Verification items for the finished model (mm, model axes). Face numbers are marked on the shaded views. Coordinates: 2 decimals unless noted, no trailing zeros. Loops run counter-clockwise (first coordinate to the right, second up) from the corner with the lowest first, then second, coordinate; pieces in that order, holes last. Notation, with made-up numbers: M 24.25,38 L 67.25,38 A31 ccw 67.25,62 Z; hole C 10.25,19.25 d6. An arc over 180 degrees is marked long. Write item = value, one per line. Start each with the question number.
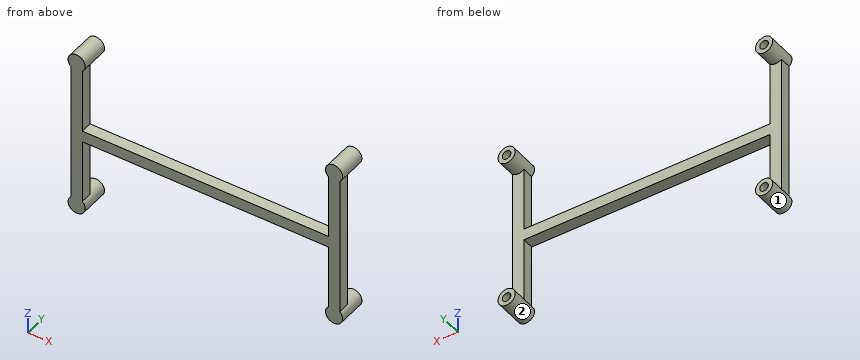
Autodesk Fusion 360 part; units mm, degrees
sketch "Schizzo9" plane through (0, 0, 0) normal (0, 1, 0) x (1, 0, 0)
  line L0 (11, 28) -> (76.9, 28)
  line L1 (76.9, 28) -> (76.9, -18)
  line L2 (76.9, -18) -> (11, -18)
  line L3 (11, -18) -> (11, 28)
  circle A0 centre (11, 28) radius 2.75
  circle A1 centre (76.9, 28) radius 2.75
  circle A2 centre (11, -18) radius 2.75
  circle A3 centre (76.9, -18) radius 2.75
  line L4 (11, 28) -> (9, 28)
  line L5 (11, 28) -> (13, 28)
  line L6 (9, 28) -> (9, -18)
  line L7 (13, 28) -> (13, -18)
  line L8 (76.9, 28) -> (74.9, 28)
  line L9 (76.9, 28) -> (78.9, 28)
  line L10 (78.9, 28) -> (78.9, -18)
  line L11 (74.9, 28) -> (74.9, -18)
  line L12 (78.9, 5) -> (78.9, 7)
  line L13 (78.9, 5) -> (78.9, 3)
  line L14 (78.9, 7) -> (9, 7)
  line L15 (78.9, 3) -> (9, 3)
  dimension "d99" = 65.9
  dimension "d100" = 46
  dimension "d101" = 5.5
  dimension "d102" = 5.5
  dimension "d103" = 5.5
  dimension "d104" = 5.5
  dimension "d105" = 2
  dimension "d106" = 2
  dimension "d107" = 2
  dimension "d108" = 2
  dimension "d109" = 2
  dimension "d110" = 2
sketch "Schizzo10" plane through (0, 0, 0) normal (0, 1, 0) x (1, 0, 0)
  line L0 (26, 54) -> (116, 54)
  line L1 (116, 54) -> (116, 0.8)
  line L2 (116, 0.8) -> (26, 0.8)
  line L3 (26, 0.8) -> (26, 54)
  circle A0 centre (26, 54) radius 3
  circle A1 centre (26, 0.8) radius 3
  circle A2 centre (116, 54) radius 3
  circle A3 centre (116, 0.8) radius 3
  line L4 (26, 54) -> (24, 54)
  line L5 (26, 54) -> (28, 54)
  line L6 (24, 54) -> (24, 0.8)
  line L7 (28, 54) -> (28, 0.8)
  line L8 (116, 54) -> (114, 54)
  line L9 (116, 54) -> (118, 54)
  line L10 (118, 54) -> (118, 0.8)
  line L11 (114, 54) -> (114, 0.8)
  line L12 (118, 27.4) -> (118, 25.4)
  line L13 (118, 27.4) -> (118, 29.4)
  line L14 (118, 29.4) -> (24, 29.4)
  line L15 (118, 25.4) -> (24, 25.4)
  dimension "d127" = 90
  dimension "d128" = 53.2
  dimension "d129" = 6
  dimension "d130" = 6
  dimension "d131" = 6
  dimension "d132" = 6
  dimension "d133" = 2
  dimension "d134" = 2
  dimension "d135" = 2
  dimension "d136" = 2
  dimension "d137" = 2
  dimension "d138" = 2
extrude "Estrusione18" add sketch "Schizzo10" along normal blind 4 contours L3 A0 L7 L14 | L3 A0 L6 L14 | L3 L7 L14 L15 | L3 L6 L14 L15 | L7 L11 L14 L15 | L3 A1 L7 L15 | L3 A1 L6 L15 | L1 A2 L11 L14 | L1 L11 L14 L15 | L1 A2 L10 L14 | L1 A3 L11 L15 | L1 L10 L12 L13 L14 L15 | L1 A3 L10 L15
extrude "Estrusione19" add sketch "Schizzo10" along normal blind 10 contours L0 A0 L4 L5 L6 | L0 L3 A0 L5 L7 | L3 A0 L4 L6 | L0 A0 L7 | L0 A2 L8 L9 L10 | L0 A2 L11 | L0 L1 A2 L8 L11 | L2 L3 A1 L7 | L2 L3 A1 | L1 A2 L9 L10 | L2 A1 L7 | L2 A3 L11 | L1 L2 A3 L11 | L1 L2 A3
hole "Foratura13" at (26, 10, -54) direction (0, -1, 0) diameter 3 depth 3 tip angle 118
hole "Foratura14" at (26, 10, -0.8) direction (0, -1, 0) diameter 3 depth 3 tip angle 118
hole "Foratura15" at (116, 10, -0.8) direction (0, -1, 0) diameter 3 depth 3 tip angle 118
hole "Foratura16" at (116, 10, -54) direction (0, -1, 0) diameter 3 depth 3 tip angle 118
Q1. Sectioned sample at A-A on y = 8. Record the cut outline in (x, z), plus the area to 3 significant figures.
Q2. Mould release check, pull along Z, two halves, no side actions. Record for the marked faces 1 and 2: +Z half, -Z half, draft (parallel to the pull), parting line (faces both ways), or undercut.
Q3. Sectioned sample at D-D on x = 35. Record the cut outline in (y, z).
Q4. Sectioned sample at C-C on y = 2.5. Record the cut outline in (x, z).
Q5. Sectioned sample at B-B on z = -31. Record the cut outline in (x, y).
Q6. Gauge pin test, flat ends, axial feed: pin 1 (24.5 mm diameter, centred on x = 63.5, z = -16.5, fed in from +Y); pin 2 (4.5 mm diameter, centred on x = 52, y = 2, fed in from +Z); pin 3 (4 mm diameter, centred on y = 2.5, z = -49.5, fed in from +X); pin 4 (2 mm diameter, centred on x = 96, z = -23, fed in from -Y). Record the tip position at first contact, or that the pin passes through.
Q7. Scan lines: L1, parallel to X at y = 8.05, z = -0.8; L2, parallel to Z at x = 116, y = 9.2; L3, parallel to X at y = 3, z = -12. Record each from-to range of solid material in increasing order. Write a range as [from, to].
Solutions:
q1.outline = C 26,-54 d6; C 26,-0.8 d6; C 116,-54 d6; C 116,-0.8 d6; hole C 26,-54 d3; hole C 26,-0.8 d3; hole C 116,-54 d3; hole C 116,-0.8 d3
q1.area = 84.8 mm²
q2.face_1 = undercut
q2.face_2 = undercut
q3.outline = M 0,-29.4 L 4,-29.4 L 4,-25.4 L 0,-25.4 Z
q4.outline = M 24,-51.76 A3 ccw long 28,-51.76 L 28,-29.4 L 114,-29.4 L 114,-51.76 A3 ccw long 118,-51.76 L 118,-3.04 A3 ccw long 114,-3.04 L 114,-25.4 L 28,-25.4 L 28,-3.04 A3 ccw long 24,-3.04 Z
q5.outline = M 24,0 L 28,0 L 28,4 L 24,4 Z; M 114,0 L 118,0 L 118,4 L 114,4 Z
q6.pin_1 = 4
q6.pin_2 = -25.4
q6.pin_3 = 118
q6.pin_4 = through
q7.L1 = [23, 24.5], [27.5, 29], [113, 114.5], [117.5, 119]
q7.L2 = [-57, -55.5], [-52.5, -51], [-3.8, -2.3], [0.7, 2.2]
q7.L3 = [24, 28], [114, 118]
